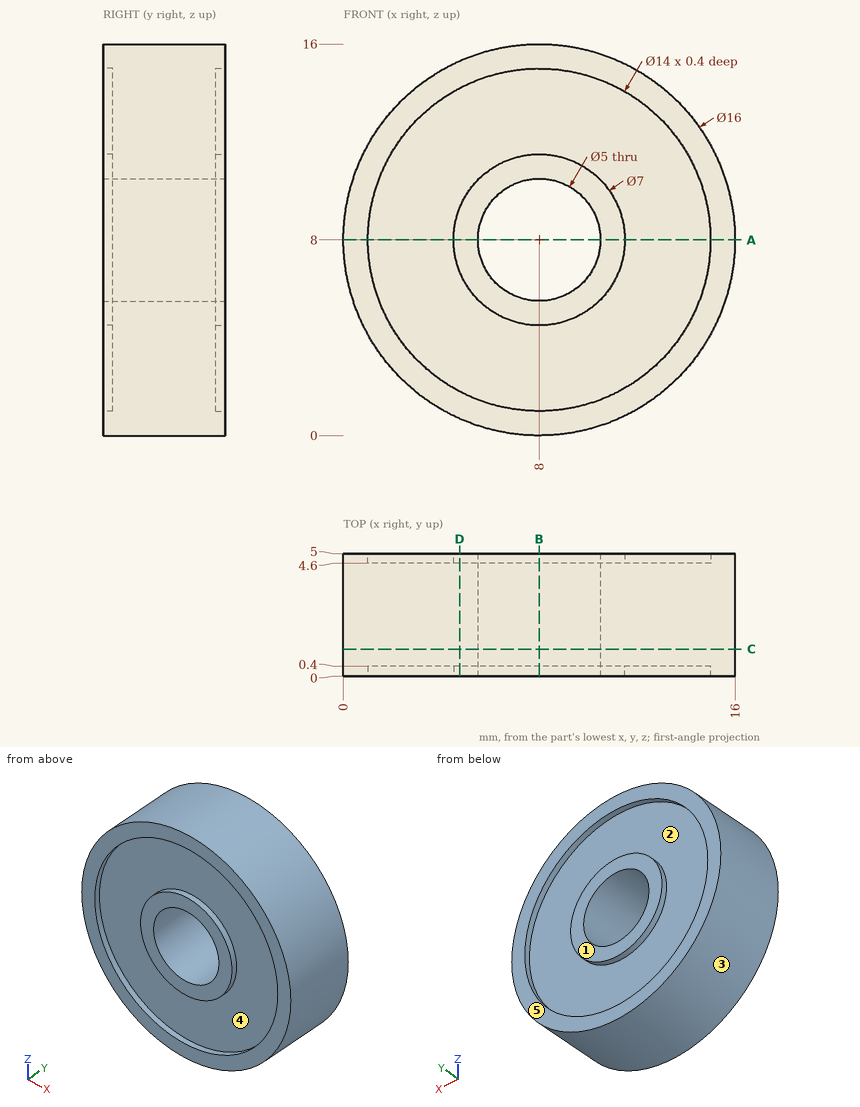
The drawing under review shows one solid part. Ordinate dimensions are in mm from its lowest x, y, z. A direction names the side the tool comes from. Coordinates: 2 decimals unless noted, no trailing zeros. Loops run counter-clockwise (first coordinate to the right, second up) from the corner with the lowest first, then second, coordinate; pieces in that order, holes last. Notation, with made-up numbers: (85.25, -29) - (128.25, -29) arc R16 cw to (128.25, -23) - close; hole circle Ø2 at (-1.75, 88). An arc over 180 degrees is marked (long way). Return JSON: item names as keys, results as strings.
Item 1: For the marked faces 4 and 5, list the 3-axis set-ups (+Z, -Z, +X, -X, +Y, -Y) from which the entire face can be reached by the end or side of a thin tool; tool diameter is ignored.
Determined:
{"face 4": "-Y", "face 5": "+Z, -Z, +X, -X, +Y"}
Item 2: Mouldability with a two-part tool opening along X and no side actions: class the marked faces 1, 2 and 3 as pulls with the +X half, pulls with the -X half, needs draft (parallel to the pull), parting line crosses it, or undercut.
Determined:
{"face 1": "needs draft", "face 2": "undercut", "face 3": "parting line crosses it"}
Item 3: Insertion check: pin 1 (4 mm diameter, centred on x = 8, z = 8, fed in from -Y); pin 2 (7 mm diameter, centred on x = 7, z = 10.5, fed in from -Y); pin 3 (3 mm diameter, centred on y = 2, z = 2.5, fed in from -X); pin 4 (1.5 mm diameter, centred on x = 4.5, z = 11, fed in from -Y). Each pin has a flat end and moves straight along its axis. Give the tip position at first contact, or say it passes through.
Determined:
{"pin 1": "passes through", "pin 2": "stops at y = 0", "pin 3": "stops at x = 1.07", "pin 4": "stops at y = 0.4"}
Item 4: Take a section at A-A (z = 8). Give the boundary of the cut face in (x, y), then the cut area to 3 significant figures.
Determined:
{"outline": "(0, 0) - (1, 0) - (1, 0.4) - (4.5, 0.4) - (4.5, 0) - (5.5, 0) - (5.5, 5) - (4.5, 5) - (4.5, 4.6) - (1, 4.6) - (1, 5) - (0, 5) - close; (10.5, 0) - (11.5, 0) - (11.5, 0.4) - (15, 0.4) - (15, 0) - (16, 0) - (16, 5) - (15, 5) - (15, 4.6) - (11.5, 4.6) - (11.5, 5) - (10.5, 5) - close", "area": "49.4 mm2"}
Item 5: For line 1 (Z direction, x = 8, y = 0.2); line 2 (Z direction, x = 8, y = 2.75), list the stretches that pass through material, from the lowest coordinate up.
Determined:
{"line 1": "z = 0 to 1, 4.5 to 5.5, 10.5 to 11.5, 15 to 16", "line 2": "z = 0 to 5.5, 10.5 to 16"}
Item 6: Take a section at C-C (y = 1.1). Give the boundary of the cut face in (x, z), then the cut area to 3 significant figures.
Determined:
{"outline": "circle Ø16 at (8, 8); hole circle Ø5 at (8, 8)", "area": "181 mm2"}
Item 7: Take a section at B-B (x = 8). Give the boundary of the cut face in (y, z).
Determined:
{"outline": "(0, 0) - (5, 0) - (5, 1) - (4.6, 1) - (4.6, 4.5) - (5, 4.5) - (5, 5.5) - (0, 5.5) - (0, 4.5) - (0.4, 4.5) - (0.4, 1) - (0, 1) - close; (0, 10.5) - (5, 10.5) - (5, 11.5) - (4.6, 11.5) - (4.6, 15) - (5, 15) - (5, 16) - (0, 16) - (0, 15) - (0.4, 15) - (0.4, 11.5) - (0, 11.5) - close"}
Item 8: Take a section at D-D (x = 4.75). Give the boundary of the cut face in (y, z).
Determined:
{"outline": "(0, 0.69) - (5, 0.69) - (5, 1.8) - (4.6, 1.8) - (4.6, 6.7) - (5, 6.7) - (5, 9.3) - (4.6, 9.3) - (4.6, 14.2) - (5, 14.2) - (5, 15.31) - (0, 15.31) - (0, 14.2) - (0.4, 14.2) - (0.4, 9.3) - (0, 9.3) - (0, 6.7) - (0.4, 6.7) - (0.4, 1.8) - (0, 1.8) - close"}
